from build123d import *

# Parameters (mm, degrees)
SKETCH1_R           = 6.4
BOSS_EXTRUDE1_DEPTH = 1.3
SKETCH1_3_R         = 5.75
BOSS_EXTRUDE2_DEPTH = 5.7
SKETCH2_W           = 5.5
SKETCH2_H           = 5.5
SKETCH2_W_2         = 3.8
SKETCH2_H_2         = 3.8
BOSS_EXTRUDE3_DEPTH = 2.5


with BuildPart() as part:
    # Sketch1 → Boss-Extrude1 (new body)
    with BuildSketch(Plane(origin=(0, 0, 0), x_dir=(1, 0, 0), z_dir=(0, 1, 0))):
        with Locations(Location((0, 0, 0), (0, 0, 270))):
            Circle(SKETCH1_R)
    extrude(amount=BOSS_EXTRUDE1_DEPTH)

    # Sketch1_3 → Boss-Extrude2 (add)
    with BuildSketch(Plane(origin=(0, 0, 0), x_dir=(1, 0, 0), z_dir=(0, 1, 0))):
        with Locations(Location((0, 0, 0), (0, 0, 270))):
            Circle(SKETCH1_3_R)
    extrude(amount=BOSS_EXTRUDE2_DEPTH)

    # Sketch2 → Boss-Extrude3 (add)
    with BuildSketch(Plane(origin=(0, 0, 0), x_dir=(1, 0, 0), z_dir=(0, 1, 0))):
        Rectangle(SKETCH2_W, SKETCH2_H)
        Rectangle(SKETCH2_W_2, SKETCH2_H_2, mode=Mode.SUBTRACT)
    extrude(amount=-BOSS_EXTRUDE3_DEPTH)


solid = part.part
Input: part model. Units: mm. Frame: model coordinates. A direction names the side the tool comes from. Round coordinates to 2 decimals unless told otherwise and drop trailing zeros. Order: outer loops, then holes, each group sorted by start corner. A loop starts at its lowest first (then second) coordinate and runs counter-clockwise, first axis right, second up. Notation, with made-up numbers: (-12.5, 43) - (42.5, 43) arc R22 cw to (42.5, 67) - close; hole circle Ø11 at (60.5, 63). An arc over 180 degrees is marked (long way). Answer as a JSON object with one key per item and string values. Group by question number.
(1) Cut plane A-A (z = 3.5). Return loops of the section in (x, y), then the cut area to 3 significant figures.
(2) Cut plane D-D (z = 0). Return loops of the section in (x, y), then the cut area to 3 significant figures.
(3) Cut plane C-C (y = 5.25). Return loops of the section in (x, z), then the cut area to 3 significant figures.
(4) Cut plane B-B (x = 0). Return loops of the section in (y, z), then the cut area to 3 significant figures.
(5) Draft query along X for faces 4 (the face through (0, -1, -1.9)), 5 (the face through (-2.75, -1, 0)), 6 (the face through (0, -1, -2.75)). Return one class per face: released by +X, released by -X, zero draft, split by the parting line, or undercut.
(6) Pin query (flat end, axial travel): P1, Ø4, axis at x = 0, z = 0.5, coming from the -Y side; P2, Ø1, axis at x = 1, y = 4.5, coming from the -Z side; P3, Ø1.2, axis at y = -1, z = 0.5, coming from the -X side; P4, Ø1.2, axis at y = -1.5, z = -0.5, coming from the +X side. Return the tip coordinate at first contact, or that it passes through.
(7) Material intervals for probe 1 along Y at (x, z) = (1.25, 1.5); probe 2 along X at (y, z) = (-0.25, 0); probe 3 along Y at (x, z) = (2.5, 5.75), sorted ascending. Write a range as from..to.
(8) Reachability of faces 1 (the face through (0, 0, 0)), 2 (the face through (2.75, -1, 0)), 3 (the face through (1, 1.3, -6)) from +Z, -Z, +X, -X, +Y, -Y: full face, straight path, thin tool, end or side. Return the list, or none.
Here are the results:
{
 "1": {"outline": "(-5.36, 0) - (5.36, 0) - (5.36, 1.3) - (4.56, 1.3) - (4.56, 5.7) - (-4.56, 5.7) - (-4.56, 1.3) - (-5.36, 1.3) - close", "area": "54.1 mm^2"},
 "2": {"outline": "(-6.4, 0) - (-2.75, 0) - (-2.75, -2.5) - (-1.9, -2.5) - (-1.9, 0) - (1.9, 0) - (1.9, -2.5) - (2.75, -2.5) - (2.75, 0) - (6.4, 0) - (6.4, 1.3) - (5.75, 1.3) - (5.75, 5.7) - (-5.75, 5.7) - (-5.75, 1.3) - (-6.4, 1.3) - close", "area": "71.5 mm^2"},
 "3": {"outline": "circle Ø11.5 at (0, 0)", "area": "104 mm^2"},
 "4": {"outline": "(-2.5, -2.75) - (0, -2.75) - (0, -6.4) - (1.3, -6.4) - (1.3, -5.75) - (5.7, -5.75) - (5.7, 5.75) - (1.3, 5.75) - (1.3, 6.4) - (0, 6.4) - (0, 2.75) - (-2.5, 2.75) - (-2.5, 1.9) - (0, 1.9) - (0, -1.9) - (-2.5, -1.9) - close", "area": "71.5 mm^2"},
 "5": {"face 4": "undercut", "face 5": "released by -X", "face 6": "zero draft"},
 "6": {"P1": "stops at y = -2.5", "P2": "stops at z = -5.73", "P3": "stops at x = -2.75", "P4": "stops at x = 2.75"},
 "7": {"probe 1": "y = 0..5.7", "probe 2": "x = -2.75..-1.9, 1.9..2.75", "probe 3": "y = 0..1.3"},
 "8": {"face 1": "-Y", "face 2": "+Z, -Z, +X, -Y", "face 3": "+Y"}
}
